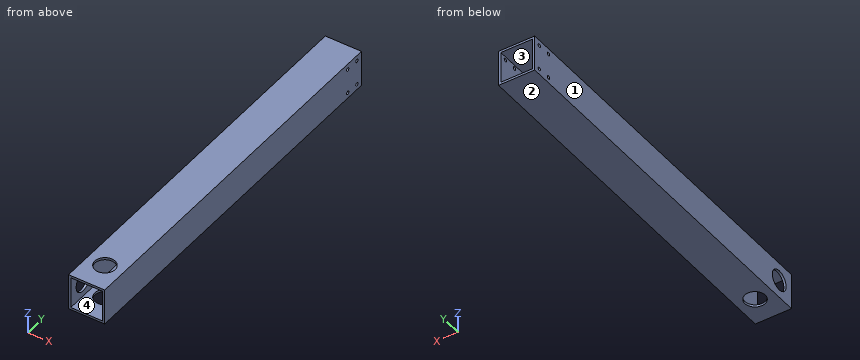
```python
from build123d import *

# Parameters (mm, degrees)
SKETCH1_W           = 50.8
SKETCH1_H           = 50.8
SKETCH1_W_2         = 44.45
SKETCH1_H_2         = 44.45
BOSS_EXTRUDE1_DEPTH = 533.4
SKETCH2_R           = 14.2875
CUT_EXTRUDE1_DEPTH  = 3.175
SKETCH3_R           = 14.3002
CUT_EXTRUDE2_DEPTH  = 537.415286881
SKETCH4_R           = 2.38125
CUT_EXTRUDE3_DEPTH  = 537.415286881


with BuildPart() as part:
    # Sketch1 → Boss-Extrude1 (new body)
    with BuildSketch(Plane(origin=(0, 0, 0), x_dir=(1, 0, 0), z_dir=(0, 1, 0))):
        Rectangle(SKETCH1_W, SKETCH1_H)
        Rectangle(SKETCH1_W_2, SKETCH1_H_2, mode=Mode.SUBTRACT)
    extrude(amount=BOSS_EXTRUDE1_DEPTH)

    # Sketch2 → Cut-Extrude1 (cut)
    with BuildSketch(Plane.ZY.offset(25.4)):
        with Locations((0, 25.4)):
            Circle(SKETCH2_R)
    extrude(amount=-CUT_EXTRUDE1_DEPTH, mode=Mode.SUBTRACT)

    # Sketch3 → Cut-Extrude2 (cut, through all)
    with BuildSketch(Plane(origin=(0, 0, -25.4), x_dir=(-1, 0, 0), z_dir=(0, 0, -1))):
        with Locations((0, 38.1)):
            Circle(SKETCH3_R)
    extrude(amount=-CUT_EXTRUDE2_DEPTH, mode=Mode.SUBTRACT)

    # Sketch4 → Cut-Extrude3 (cut, through all)
    with BuildSketch(Plane.ZY.offset(25.4)):
        with Locations((17.4625, 523.875)):
            Circle(SKETCH4_R)
        with Locations((17.4625, 504.825)):
            Circle(SKETCH4_R)
        with Locations((-17.4625, 504.825)):
            Circle(SKETCH4_R)
        with Locations((-17.4625, 523.875)):
            Circle(SKETCH4_R)
    extrude(amount=-CUT_EXTRUDE3_DEPTH, mode=Mode.SUBTRACT)


solid = part.part
```
Geometry check sheet. Reference: the model listing, model coordinates, mm. Face numbers are marked on the shaded views. Coordinates: 2 decimals unless noted, no trailing zeros. Order: outer loops, then holes, each group sorted by start corner. A loop starts at its lowest first (then second) coordinate and runs counter-clockwise, first axis right, second up.
Item 1: Section check C-C (z = 0). Enter the section's corners in (x, y) (1 decimal), plus the area to 3 significant figures.
Item 2: Mould release check, pull along X, two halves, no side actions. Record for the marked faces 1, 2, 3 and 4: released by +X, released by -X, zero draft, split by the parting line, or undercut.
Item 3: Section check B-B (y = 310). Enter the section's corners in (x, z) (3 decimals), plus the area to 3 significant figures.
Item 4: Scan lines: line 1 along Y through (x, z) = (-23.75, 0); line 2 along X through (y, z) = (73, -21) (3 decimals). Record each from-to range of solid material in increasing order.
Item 5: Section check A-A (x = 0). Enter the section's corners in (y, z) (3 decimals), plus the area to 3 significant figures.
Item 6: Depth check by flat-ended pin: pin 1 (5 mm diameter, centred on x = 19, z = -7, fed in from -Y); pin 2 (6 mm diameter, centred on y = 523.88, z = -17.46, fed in from +X). Enter the tip coordinate at first touch or a pass-through.
Check sheet entries:
1. outline: (-25.4, 0) - (-22.2, 0) - (-22.2, 11.1) - (-25.4, 11.1) - close; (-25.4, 39.7) - (-22.2, 39.7) - (-22.2, 533.4) - (-25.4, 533.4) - close; (22.2, 0) - (25.4, 0) - (25.4, 533.4) - (22.2, 533.4) - close
1. area: 3,300 mm2
2. face 1: released by -X
2. face 2: zero draft
2. face 3: undercut
2. face 4: undercut
3. outline: (-25.4, -25.4) - (25.4, -25.4) - (25.4, 25.4) - (-25.4, 25.4) - close; hole (-22.225, -22.225) - (22.225, -22.225) - (22.225, 22.225) - (-22.225, 22.225) - close
3. area: 605 mm2
4. line 1: y = 0 to 11.11, 39.69 to 533.4
4. line 2: x = -25.4 to -22.225, 22.225 to 25.4
5. outline: (0, -25.4) - (23.8, -25.4) - (23.8, -22.225) - (0, -22.225) - close; (0, 22.225) - (23.8, 22.225) - (23.8, 25.4) - (0, 25.4) - close; (52.4, -25.4) - (533.4, -25.4) - (533.4, -22.225) - (52.4, -22.225) - close; (52.4, 22.225) - (533.4, 22.225) - (533.4, 25.4) - (52.4, 25.4) - close
5. area: 3,210 mm2
6. pin 1: passes through
6. pin 2: stops at x = 25.4
